Could you check a few things on this model? Use its own coordinates, in mm. A direction names the side the tool comes from. Round coordinates to 2 decimals unless told otherwise and drop trailing zeros. Write each loop counter-clockwise with the first axis right and the second up, starting at its lowest first coordinate (ties: lowest second). Pieces come first, ordered by that corner, then holes. Notation, with made-up numbers: (50, 57) -> (83, 57) arc R21 ccw to (83, 61) -> close; hole circle Ø6 at (6, -36). An arc over 180 degrees is marked (long way). One line per question, with ' | ' between items. Start each with the question number.
1. Imagine slicing it at B-B, the plane x = 0. List the corners of the cut face in (y, z) for me.
2. For pin 1 Ø16 at (x, y) = (-71.5, -0.5) entering from +Z; pin 2 Ø2 at (x, z) = (-11.5, 14.5) entering from +Y; pin 3 Ø6 at (x, y) = (-65.5, 11) entering from +Z, each with a flat end and sliding along its axis, tell me the tip position at first contact or that it passes through.
3. For faces 1 (the flat face through (-39.28, -13.392, -0.07)), 2 (the flat face through (-80, -2, 6)), 3 (the flat face through (-11, -3, 7)), which set-ups out of +Z, -Z, +X, -X, +Y, -Y let a thin tool reach every point of the face, with its end or its side?
4. Thinking about a two-plate mould opening in X: for faces 4 (the flat face through (-80, -2, -6)), 5 (the flat face through (-38.24, 13.49, 0.07)), 6 (the flat face through (-13, 0, 7)), 7 (the flat face through (-11, 3, 7)), which applies, released by +X, released by -X, zero draft, split by the parting line, or undercut?
5. Imagine slicing it at C-C, the plane z = -1.5. List the corners of the cut face in (x, y) for me.
6. If I drill on line 1 along Y through (x, z) = (0, 8.5); line 2 along X through (y, z) = (0.5, -4); line 3 along X through (y, z) = (-3.5, 1.5), over which ranges is the centre line in solid material (lowest first)? Write a range as [from, to].
7. Imagine slicing it at A-A, the plane y = 0. List the corners of the cut face in (x, z) for me, and give its area (3 significant figures).
8. Imagine slicing it at D-D, the plane y = 9. List the corners of the cut face in (x, z) for me, and give its area (3 significant figures).
from build123d import *

# Parameters (mm, degrees)
SCHIZZO2_R                        = 10
ESTRUSIONE_ESTRUSIONE1_DEPTH      = 6
ESTRUSIONE_ESTRUSIONE2_DEPTH      = 21
ESTRUSIONE_ESTRUSIONE2_DEPTH_BACK = 6
SCHIZZO2_3_R                      = 17
ESTRUSIONE_ESTRUSIONE3_DEPTH      = 5
FORO_10_0_10_1_D                  = 10


with BuildPart() as part:
    # Schizzo2 → Estrusione-Estrusione1 (new, symmetric)
    with BuildSketch(Plane.XY):
        with Locations((-75, 0)):
            Circle(SCHIZZO2_R)
    extrude(amount=ESTRUSIONE_ESTRUSIONE1_DEPTH, both=True)



with BuildPart() as body_2:
    # Schizzo2_3 → Estrusione-Estrusione2 (new, two sides: drawn at the far end of the back side and taken through both)
    with BuildSketch(Plane.XY.offset(-ESTRUSIONE_ESTRUSIONE2_DEPTH_BACK)):
        Circle(SCHIZZO2_3_R)
        with BuildLine():
            Line((-13, 3), (-9.539392014, 3))
            ThreePointArc((-9.539392014, 3), (10, 0), (-9.539392014, -3))
            Line((-9.539392014, -3), (-13, -3))
            Line((-13, -3), (-13, 3))
        make_face(mode=Mode.SUBTRACT)
    extrude(amount=ESTRUSIONE_ESTRUSIONE2_DEPTH + ESTRUSIONE_ESTRUSIONE2_DEPTH_BACK)


with BuildPart() as part_1:
    add(part.part)

    add(body_2.part)  # Estrusione-Estrusione3 merges body 2
    # Schizzo2_4 → Estrusione-Estrusione3 (add, symmetric)
    with BuildSketch(Plane.XY):
        with BuildLine():
            ThreePointArc((-75.933333333, 9.956349175), (-68.266996708, 7.393691004), (-65, 0))
            Line((-65, 0), (-17, 0))
            ThreePointArc((-17, 0), (-12.569274707, 11.446105597), (-1.586666667, 16.925793597))
            Line((-1.586666667, 16.925793597), (-75.933333333, 9.956349175))
        make_face()
        with BuildLine():
            Line((-17, 0), (-65, 0))
            ThreePointArc((-65, 0), (-68.266996708, -7.393691004), (-75.933333333, -9.956349175))
            Line((-75.933333333, -9.956349175), (-1.586666667, -16.925793597))
            ThreePointArc((-1.586666667, -16.925793597), (-12.569274707, -11.446105597), (-17, 0))
        make_face()
    extrude(amount=ESTRUSIONE_ESTRUSIONE3_DEPTH, both=True)

    # Foro _10.0 _10_-1 (through all)
    with Locations(Plane.XY.offset(6)):
        with Locations((-75, 0)):
            Hole(FORO_10_0_10_1_D / 2)


solid = part_1.part
Geometry results:
1) outline: (-17, -6) -> (-10, -6) -> (-10, 21) -> (-17, 21) -> close; (10, -6) -> (17, -6) -> (17, 21) -> (10, 21) -> close
2) pin 1: stops at z = 6 | pin 2: stops at y = 13.37 | pin 3: stops at z = 5
3) face 1: +Z, -Z, -X, -Y | face 2: +Z, -X, +Y, -Y | face 3: +Z, -Z
4) face 4: zero draft | face 5: released by -X | face 6: undercut | face 7: undercut
5) outline: (-75.93, -9.96) -> (-1.59, -16.93) arc R17 ccw (long way) to (-1.59, 16.93) -> (-75.93, 9.96) arc R10 ccw to start; hole circle Ø10 at (-75, 0); hole (-13, -3) -> (-9.54, -3) arc R10 ccw (long way) to (-9.54, 3) -> (-13, 3) -> close
6) line 1: y = [-17, -10], [10, 17] | line 2: x = [-84.99, -79.97], [-70.03, -13], [9.99, 16.99] | line 3: x = [-84.37, -78.57], [-71.43, -9.37], [9.37, 16.64]
7) outline: (-85, -6) -> (-80, -6) -> (-80, 6) -> (-85, 6) -> close; (-70, -6) -> (-65, -6) -> (-65, -5) -> (-17, -5) -> (-17, -6) -> (-13, -6) -> (-13, 21) -> (-17, 21) -> (-17, 5) -> (-65, 5) -> (-65, 6) -> (-70, 6) -> close; (10, -6) -> (17, -6) -> (17, 21) -> (10, 21) -> close | area: 897 mm2
8) outline: (-79.36, -6) -> (-70.64, -6) -> (-70.64, -5) -> (-14.42, -5) -> (-14.42, -6) -> (-4.36, -6) -> (-4.36, 21) -> (-14.42, 21) -> (-14.42, 5) -> (-70.64, 5) -> (-70.64, 6) -> (-79.36, 6) -> close; (4.36, -6) -> (14.42, -6) -> (14.42, 21) -> (4.36, 21) -> close | area: 1,210 mm2
